Design review of the part built by this model. Coordinates are the model's own, in mm. Give positions to 0.01 mm unless a question says otherwise; leave off trailing zeros. Loops run counter-clockwise (first coordinate to the right, second up) from the corner with the lowest first, then second, coordinate; pieces in that order, holes last. Notation, with made-up numbers: (-2, -5) -> (41, -5) arc R24 ccw to (41, 30) -> close; hole circle Ø5 at (-17, 6). An arc over 180 degrees is marked (long way). Use a Markdown table: item, result. Add a question column.
1. Add section A-A (y = 62). State the section outline as (x, z) points.
2. Add section C-C (x = 71.8). State the section outline as (y, z) points.
3. Add section B-B (z = 26.9). State the section outline as (x, y) points.
4. To check wall thickness, follow line 1 (X direction, y = 56.5, z = 26.75); line 2 (Z direction, x = 72.2, y = 79); line 3 (Z direction, x = 73, y = 46). State the ranges of each line that lie inside material, in increasing order.
5. For pin 1 Ø1 at (x, y) = (72.5, 22) entering from -Z; pin 2 Ø0.7 at (y, z) = (33, 26) entering from +X, all flat-tipped, find the tip position at first contact; note any pin that passes through.
```python
from build123d import *

# Parameters (mm, degrees)
EXTRUDE104_DEPTH                  = 81.5
PART_MIRRORING002_PLACEMENT_ANGLE = 90


with BuildPart() as bottom_notch003:
    # Sketch106 → Extrude104 (new body)
    with BuildSketch(Plane.YZ):
        Polygon((1.890375, 25.594459), (1.890375, 27.613628), (1.890375, 28.007893), (1.285825, 28.007893), (1.394986, 27.535334), (0.819798, 27.769814), (0.819798, 28.652969), (2.608973, 28.652969), (2.608973, 26.491592), align=None)
    extrude(amount=EXTRUDE104_DEPTH)


with BuildPart() as bottom_notch003_1:
    # Extrude104 placement: moved
    add(bottom_notch003.part.moved(Location((4.5, 0, -0.1))))


with BuildPart() as right_notch:
    # Part__Mirroring002: instance of Bottom_Notch003
    add(bottom_notch003_1.part.mirror(Plane(origin=(37, 2e-06, 27.023727), x_dir=(1, 0, 0), z_dir=(0, 1, 0))))


with BuildPart() as right_notch_1:
    # Part__Mirroring002 placement: moved
    add(right_notch.part.rotate(Axis((0, 0, 0), (0, 0, 1)), PART_MIRRORING002_PLACEMENT_ANGLE))


with BuildPart() as part_mirroring003:
    # Part__Mirroring003: instance of right_notch
    add(right_notch_1.part.mirror(Plane(origin=(0, 0, 0), x_dir=(0, -1, 0), z_dir=(1, 0, 0))))


with BuildPart() as part_mirroring003_1:
    # Part__Mirroring003 placement: moved
    add(part_mirroring003.part.moved(Location((74, 0, 0))))


solid = part_mirroring003_1.part
```
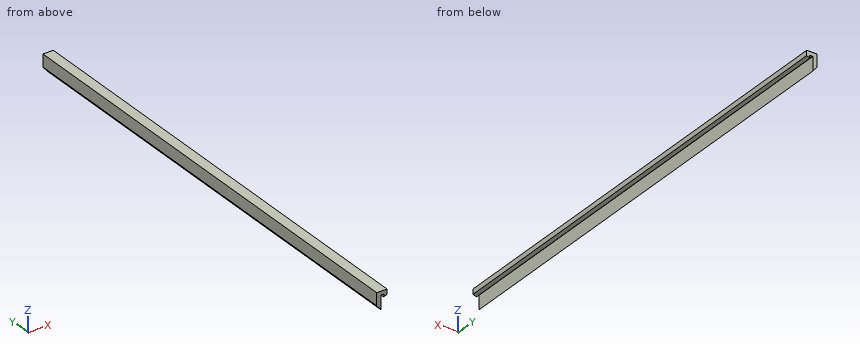
Taken from the geometry:
| question | item | result |
|---|---|---|
| 1 | outline | (71.39, 26.39) -> (72.11, 25.49) -> (72.11, 27.91) -> (72.71, 27.91) -> (72.61, 27.44) -> (73.18, 27.67) -> (73.18, 28.55) -> (71.39, 28.55) -> close |
| 2 | outline | (4.5, 25.88) -> (86, 25.88) -> (86, 28.55) -> (4.5, 28.55) -> close |
| 3 | outline | (71.39, 4.5) -> (72.11, 4.5) -> (72.11, 86) -> (71.39, 86) -> close |
| 4 | line 1 | x = 71.39 to 72.11 |
| 4 | line 2 | z = 27.91 to 28.55 |
| 4 | line 3 | z = 27.6 to 28.55 |
| 5 | pin 1 | stops at z = 25.49 |
| 5 | pin 2 | stops at x = 72.11 |
